```python
from build123d import *

# Parameters (mm, degrees)
ESQUISSE1_W                  = 55
ESQUISSE1_H                  = 45
BOSS_EXTRU_1_DEPTH           = 12
ESQUISSE2_R                  = 4.25
ENL_V_MAT_EXTRU_1_DEPTH      = 55.085580333
ENL_V_MAT_EXTRU_2_DEPTH      = 12.25
ENL_V_MAT_EXTRU_2_DEPTH_BACK = 12.25
ESQUISSE3_R                  = 7.75
ESQUISSE4_R                  = 11
ENL_V_MAT_EXTRU_3_DEPTH      = 3
ESQUISSE5_R                  = 5
ENL_V_MAT_EXTRU_4_DEPTH      = 15
ENL_V_MAT_EXTRU_5_DEPTH      = 38.503333185
ENL_V_MAT_EXTRU_5_DEPTH_BACK = 38.503333185
ESQUISSE6_R                  = 1.5
ESQUISSE7_R                  = 2.5
ENL_V_MAT_EXTRU_6_DEPTH      = 4
CHANFREIN3_SIZE              = 5
ESQUISSE9_W                  = 60
ESQUISSE9_H                  = 18
BOSS_EXTRU_2_DEPTH           = 27
ESQUISSE10_W                 = 41.5
ESQUISSE10_H                 = 22
ENL_V_MAT_EXTRU_7_DEPTH      = 30
ESQUISSE11_R                 = 2.15
ENL_V_MAT_EXTRU_8_DEPTH      = 52.198144498
CONG_2_R                     = 5
CONG_3_R                     = 5
ESQUISSE12_W                 = 5
ESQUISSE12_H                 = 2
ENL_V_MAT_EXTRU_9_DEPTH      = 9
SYM_TRIE4_COPY_1_SKETCH_W    = 5
SYM_TRIE4_COPY_1_SKETCH_H    = 2
SYM_TRIE4_COPY_1_DEPTH       = 9
ESQUISSE13_W                 = 29
ESQUISSE13_H                 = 3
BOSS_EXTRU_3_DEPTH           = 27
BOSS_EXTRU_4_REACH           = 53.198
ESQUISSE14_W                 = 29
ESQUISSE14_H                 = 2.5
ESQUISSE15_R                 = 1.5
ENL_V_MAT_EXTRU_10_DEPTH     = 9
ENL_V_MAT_EXTRU_11_DEPTH     = 2


with BuildPart() as part:
    # Esquisse1 → Boss.-Extru.1 (new body)
    with BuildSketch(Plane.XY):
        Rectangle(ESQUISSE1_W, ESQUISSE1_H)
    extrude(amount=BOSS_EXTRU_1_DEPTH)

    # Esquisse2 → Enlèv. mat.-Extru.1 (cut, through all)
    with BuildSketch(Plane(origin=(0, 22.5, 0), x_dir=(1, 0, 0), z_dir=(0, 1, 0))):
        with Locations((-12.5, -12)):
            Circle(ESQUISSE2_R)
        with Locations((12.5, -12)):
            Circle(ESQUISSE2_R)
    extrude(amount=-ENL_V_MAT_EXTRU_1_DEPTH, mode=Mode.SUBTRACT)

    # Esquisse3 → Enlèv. mat.-Extru.2 (cut, two sides: drawn at the far end of the back side and taken through both)
    with BuildSketch(Plane(origin=(0, 0, 0), x_dir=(1, 0, 0), z_dir=(0, 1, 0)).offset(-ENL_V_MAT_EXTRU_2_DEPTH_BACK)):
        with Locations((-12.5, -12)):
            Circle(ESQUISSE3_R)
    extrude(amount=ENL_V_MAT_EXTRU_2_DEPTH + ENL_V_MAT_EXTRU_2_DEPTH_BACK, mode=Mode.SUBTRACT)

    # Esquisse4 → Enlèv. mat.-Extru.3 (cut)
    with BuildSketch(Plane(origin=(0, 7.5, 0), x_dir=(1, 0, 0), z_dir=(0, 1, 0))):
        with Locations((12.5, -12)):
            Circle(ESQUISSE4_R)
    enl_v_mat_extru_3 = extrude(amount=-ENL_V_MAT_EXTRU_3_DEPTH, mode=Mode.SUBTRACT)

    # Esquisse5 → Enlèv. mat.-Extru.4 (cut)
    with BuildSketch(Plane(origin=(0, 7.5, 0), x_dir=(1, 0, 0), z_dir=(0, 1, 0))):
        with Locations((12.5, -12)):
            Circle(ESQUISSE5_R)
    extrude(amount=-ENL_V_MAT_EXTRU_4_DEPTH, mode=Mode.SUBTRACT)

    # Esquisse6 → Enlèv. mat.-Extru.5 (cut, two sides: drawn at the far end of the back side and taken through both)
    with BuildSketch(Plane(origin=(0, 0, 0), x_dir=(-1, 0, 0), z_dir=(0, 0, -1)).offset(-ENL_V_MAT_EXTRU_5_DEPTH_BACK)):
        with Locations((23.5, -18.5)):
            Circle(ESQUISSE6_R)
        with Locations((-23.5, -18.5)):
            Circle(ESQUISSE6_R)
        with Locations((-23.5, 18.5)):
            Circle(ESQUISSE6_R)
        with Locations((23.5, 18.5)):
            Circle(ESQUISSE6_R)
    extrude(amount=ENL_V_MAT_EXTRU_5_DEPTH + ENL_V_MAT_EXTRU_5_DEPTH_BACK, mode=Mode.SUBTRACT)

    # Esquisse7 → Enlèv. mat.-Extru.6 (cut)
    with BuildSketch(Plane(origin=(0, 0, 0), x_dir=(-1, 0, 0), z_dir=(0, 0, -1))):
        with Locations((23.5, -18.5)):
            Circle(ESQUISSE7_R)
        with Locations(Location((23.5, 18.5, 0), (0, 0, 180))):
            Circle(ESQUISSE7_R)
        with Locations((-23.5, 18.5)):
            Circle(ESQUISSE7_R)
        with Locations(Location((-23.5, -18.5, 0), (0, 0, 180))):
            Circle(ESQUISSE7_R)
    extrude(amount=-ENL_V_MAT_EXTRU_6_DEPTH, mode=Mode.SUBTRACT)

    # Chanfrein3
    # the kernel refuses this chamfer: 5 mm, written as the material it takes off along each edge
    with BuildSketch(Plane(origin=(-27.5, 35.35841494, 0), x_dir=(0.9996219169112968, 0, -0.027495876610586372), z_dir=(0, -1, 0)), Plane(origin=(27.5, -35.35841494, 0), x_dir=(-0.9996219169112968, 0, -0.027495876610586372), z_dir=(0, 1, 0))) as chanfrein3_piece_1:
        Polygon((CHANFREIN3_SIZE * 0.999621916911, CHANFREIN3_SIZE * 0.0274958766106), (-CHANFREIN3_SIZE * 0.0274958766106, CHANFREIN3_SIZE * 0.999621916911), (0, 0), align=None)
    extrude(amount=70.71682988, mode=Mode.SUBTRACT)

    # Symétrie2: Enlèv. mat.-Extru.3 across plane
    add(enl_v_mat_extru_3.mirror(Plane.ZX), mode=Mode.SUBTRACT)

    # Esquisse9 → Boss.-Extru.2 (add)
    with BuildSketch(Plane(origin=(0, 0, 0), x_dir=(-1, 0, 0), z_dir=(0, 0, -1))):
        Rectangle(ESQUISSE9_W, ESQUISSE9_H)
    extrude(amount=BOSS_EXTRU_2_DEPTH)

    # Esquisse10 → Enlèv. mat.-Extru.7 (cut)
    with BuildSketch(Plane(origin=(0, 9, 0), x_dir=(1, 0, 0), z_dir=(0, 1, 0))):
        with Locations((0, 13.5)):
            Rectangle(ESQUISSE10_W, ESQUISSE10_H)
    extrude(amount=-ENL_V_MAT_EXTRU_7_DEPTH, mode=Mode.SUBTRACT)

    # Esquisse11 → Enlèv. mat.-Extru.8 (cut, through all)
    with BuildSketch(Plane(origin=(0, -9, 0), x_dir=(-1, 0, 0), z_dir=(0, -1, 0))):
        with Locations(Location((-23.15, 8.4, 0), (0, 0, 90))):
            Circle(ESQUISSE11_R)
        with Locations(Location((-23.15, 18.6, 0), (0, 0, 90))):
            Circle(ESQUISSE11_R)
        with Locations(Location((24.65, 8.4, 0), (0, 0, 90))):
            Circle(ESQUISSE11_R)
        with Locations(Location((24.65, 18.6, 0), (0, 0, 90))):
            Circle(ESQUISSE11_R)
    extrude(amount=-ENL_V_MAT_EXTRU_8_DEPTH, mode=Mode.SUBTRACT)

    # Congé2
    cong_2_edges = [part.edges().sort_by_distance(p)[0] for p in [
        (-30, 0, 0),
        (30, 0, 0),
    ]]
    fillet(cong_2_edges, radius=CONG_2_R)

    # Congé3
    cong_3_edges = [part.edges().sort_by_distance(p)[0] for p in [
        (-30, 0, -27),
        (30, 0, -27),
    ]]
    fillet(cong_3_edges, radius=CONG_3_R)

    # Esquisse12 → Enlèv. mat.-Extru.9 (cut)
    with BuildSketch(Plane(origin=(30, 0, 0), x_dir=(0, 0, -1), z_dir=(1, 0, 0))):
        with Locations((8.4, 4.5)):
            Rectangle(ESQUISSE12_W, ESQUISSE12_H)
        with Locations((18.6, 4.5)):
            Rectangle(ESQUISSE12_W, ESQUISSE12_H)
    enl_v_mat_extru_9 = extrude(amount=-ENL_V_MAT_EXTRU_9_DEPTH, mode=Mode.SUBTRACT)

    # Symétrie3: Enlèv. mat.-Extru.9 across plane
    add(enl_v_mat_extru_9.mirror(Plane(origin=(0, 0, 0), x_dir=(0, 0, 1), z_dir=(1, 0, 0))), mode=Mode.SUBTRACT)

    # Symétrie4: Enlèv. mat.-Extru.9 across plane
    add(enl_v_mat_extru_9.mirror(Plane.ZX), mode=Mode.SUBTRACT)

    # Symétrie4 copy 1 sketch → Symétrie4 copy 1 (cut)
    with BuildSketch(Plane(origin=(-30, 0, 0), x_dir=(0, 0, -1), z_dir=(-1, 0, 0))):
        with Locations((8.4, 4.5)):
            Rectangle(SYM_TRIE4_COPY_1_SKETCH_W, SYM_TRIE4_COPY_1_SKETCH_H)
        with Locations((18.6, 4.5)):
            Rectangle(SYM_TRIE4_COPY_1_SKETCH_W, SYM_TRIE4_COPY_1_SKETCH_H)
    extrude(amount=-SYM_TRIE4_COPY_1_DEPTH, mode=Mode.SUBTRACT)

    # Esquisse13 → Boss.-Extru.3 (add)
    with BuildSketch(Plane(origin=(0, 0, 0), x_dir=(-1, 0, 0), z_dir=(0, 0, -1))):
        with Locations((0, 21)):
            Rectangle(ESQUISSE13_W, ESQUISSE13_H)
    extrude(amount=BOSS_EXTRU_3_DEPTH)

    # Esquisse14 → Boss.-Extru.4 (add, up to next)
    with BuildSketch(Plane(origin=(0, 9, 0), x_dir=(1, 0, 0), z_dir=(0, 1, 0)), mode=Mode.PRIVATE) as boss_extru_4_sk1:
        with Locations((0, 25.75)):
            Rectangle(ESQUISSE14_W, ESQUISSE14_H)
    boss_extru_4_tool1 = extrude(boss_extru_4_sk1.sketch, amount=BOSS_EXTRU_4_REACH, mode=Mode.PRIVATE) - part.part
    add(boss_extru_4_tool1.solids().sort_by_distance((0, 9, -25.75))[0])

    # Esquisse15 → Enlèv. mat.-Extru.10 (cut)
    with BuildSketch(Plane(origin=(0, 22.5, 0), x_dir=(1, 0, 0), z_dir=(0, 1, 0))):
        with Locations(Location((-10.75, 13.5, 0), (0, 0, 270))):
            Circle(ESQUISSE15_R)
    extrude(amount=-ENL_V_MAT_EXTRU_10_DEPTH, mode=Mode.SUBTRACT)

    # Esquisse16 → Enlèv. mat.-Extru.11 (cut)
    with BuildSketch(Plane(origin=(0, 22.5, 0), x_dir=(1, 0, 0), z_dir=(0, 1, 0))):
        Polygon((-9.306624327, 16), (-12.193375673, 16), (-13.636751346, 13.5), (-12.193375673, 11), (-9.306624327, 11), (-7.863248654, 13.5), align=None)
    extrude(amount=-ENL_V_MAT_EXTRU_11_DEPTH, mode=Mode.SUBTRACT)


solid = part.part
```
The model under review builds one solid part; all positions refer to its coordinate system, in mm. A direction names the side the tool comes from. Give positions to 0.01 mm unless a question says otherwise; leave off trailing zeros. Write each loop counter-clockwise with the first axis right and the second up, starting at its lowest first coordinate (ties: lowest second). Pieces come first, ordered by that corner, then holes. Notation, with made-up numbers: M 39,-10 L 70,-10 A14 cw 70,7 Z; hole C -33.75,13 d6. An arc over 180 degrees is marked long. Answer in a Markdown table with one row per item.
Item 1: For P1, Ø1.5, axis at x = -27.5, z = -9.5, coming from the -Y side; P2, Ø1.5, axis at x = -25, z = -7.5, coming from the +Y side; P3, Ø1, axis at x = -7.5, z = -18.5, coming from the -Y side; P4, Ø5.5, axis at y = -2, z = 9.5, coming from the +X side, all flat-tipped, find the tip position at first contact; note any pin that passes through.
Check sheet entries:
| item | result |
|---|---|
| P1 | y = -9 |
| P2 | through |
| P3 | y = 19.5 |
| P4 | x = 27.5 |
Item 2: Add section B-B on x = -10.75. Give the boundary of the cut face in (y, z), plus the area to 3 significant figures.
Check sheet entries:
| item | result |
|---|---|
| outline | M -22.5,0 L -9,0 L -9,-2.5 L 9,-2.5 L 9,0 L 19.5,0 L 19.5,-12 L 20.5,-12 L 20.5,-11 L 22.5,-11 L 22.5,8.13 L 12.25,8.13 L 12.25,4.45 L -12.25,4.45 L -12.25,8.13 L -22.5,8.13 Z; M -9,-27 L 22.5,-27 L 22.5,-16 L 20.5,-16 L 20.5,-15 L 19.5,-15 L 19.5,-24.5 L -9,-24.5 Z |
| area | 460 mm2 |
Item 3: Add section C-C on z = -3.5. Give the boundary of the cut face in (x, y).
Check sheet entries:
| item | result |
|---|---|
| outline | M -29.77,-9 L -20.75,-9 L -20.75,9 L -29.77,9 Z; M -14.5,19.5 L 14.5,19.5 L 14.5,22.5 L -14.5,22.5 Z; M 20.75,-9 L 29.77,-9 L 29.77,9 L 20.75,9 Z |
Item 4: Draft analysis for pull direction Y (two halves, no side actions). For faces 5 (the face through (0, 0, 12)), 6 (the face through (-26, -4, -10.9)), 7 (the face through (26, -4, -21.1)), 8 (the face through (0, -22.5, 6)), state which applies: +Y half, -Y half, draft (parallel to the pull), parting line (faces both ways), or undercut.
Check sheet entries:
| item | result |
|---|---|
| face 5 | draft |
| face 6 | undercut |
| face 7 | undercut |
| face 8 | -Y half |
Item 5: Tool access review of faces 1 (the face through (21.115, 19.251, 2.416)), 2 (the face through (12.6, 0.1, 7)), 3 (the face through (-27, -3.5, -7)), 4 (the face through (-29, 0, -2)): name each direction out of +Z, -Z, +X, -X, +Y, -Y from which nothing blocks a thin tool from reaching the whole face with its end or side.
Check sheet entries:
| item | result |
|---|---|
| face 1 | -Z |
| face 2 | +Z |
| face 3 | -X |
| face 4 | -X, +Y, -Y |
Item 6: For line 1 along X through (y, z) = (2, -18.6); line 2 along Y through (x, z) = (23.5, 6.5); line 3 along Y through (x, z) = (22, 2), list the stretches that pass through material, from the lowest coordinate up.
Check sheet entries:
| item | result |
|---|---|
| line 1 | -30 to -26.8, -22.5 to -20.75, 20.75 to 21, 25.3 to 30 |
| line 2 | -22.5 to -20, -17 to 17, 20 to 22.5 |
| line 3 | -22.5 to -20.5, -16.5 to 16.5, 20.5 to 22.5 |
Item 7: Add section A-A on y = -18.5. Give the boundary of the cut face in (x, z).
Check sheet entries:
| item | result |
|---|---|
| outline | M -27.5,5 L -26,3.5 L -26,4 L -25,4 L -25,12 L -27.5,12 Z; M -22,4 L -21,4 L -21,0 L 21,0 L 21,4 L 22,4 L 22,12 L 16.75,12 A4.25 cw 8.25,12 L -8.25,12 A4.25 cw -16.75,12 L -22,12 Z; M 25,4 L 26,4 L 26,3.5 L 27.5,5 L 27.5,12 L 25,12 Z |
Item 8: Add section D-D on y = 0.5. Give the boundary of the cut face in (x, z), plus the area to 3 significant figures.
Check sheet entries:
| item | result |
|---|---|
| outline | M -30,-22 A5 ccw -25,-27 L 25,-27 A5 ccw 30,-22 L 30,-5 A5 ccw 25,0 L 22.5,0 L 27.5,5 L 27.5,12 L 17.5,12 A5 cw 7.5,12 L -4.75,12 A7.75 cw -20.25,12 L -27.5,12 L -27.5,5 L -22.5,0 L -25,0 A5 ccw -30,-5 Z; hole C -24.65,-18.6 d4.3; hole C -24.65,-8.4 d4.3; hole M -20.75,-24.5 L 20.75,-24.5 L 20.75,-2.5 L -20.75,-2.5 Z; hole C 23.15,-18.6 d4.3; hole C 23.15,-8.4 d4.3 |
| area | 1,130 mm2 |
